from build123d import *

# Parameters (mm, degrees)
F0_W     = 90
F0_H     = 40
F1_DEPTH = 90
F2_ANGLE = 90
F3_W     = 86
F3_H     = 20
F4_DEPTH = 40.001
F5_W     = 36
F5_H     = 20
F6_DEPTH = 90.001


# Not quite as in the source:
# - a feature names something its author has since deleted; it is built from what else it names


with BuildPart() as f1:
    # F0 (on Top) → F1 (new body)
    with BuildSketch(Plane.XY):
        with Locations((-1.7447127029, -1.7198646705)):
            Rectangle(F0_W, F0_H)
    extrude(amount=F1_DEPTH)


with BuildPart() as f1_1:
    # F2: moved
    add(f1.part.rotate(Axis((43.2552872971, 18.2801353295, 45), (0, 0, -1)), F2_ANGLE))

    # F3 (on face) → F4 (cut, through all)
    with BuildSketch(Plane.YZ.offset(43.2552872971)):
        with Locations((63.2801353295, 78)):
            Rectangle(F3_W, F3_H)
        with Locations((63.2801353295, 56)):
            Rectangle(F3_W, F3_H)
        with Locations((63.2801353295, 34)):
            Rectangle(F3_W, F3_H)
        with Locations((63.2801353295, 12)):
            Rectangle(F3_W, F3_H)
    extrude(amount=-F4_DEPTH, mode=Mode.SUBTRACT)

    # F5 (on face) → F6 (cut, through all)
    with BuildSketch(Plane.XZ.offset(-18.2801353295)):
        with Locations((23.2552872971, 78)):
            Rectangle(F5_W, F5_H)
        with Locations((23.2552872971, 56)):
            Rectangle(F5_W, F5_H)
        with Locations((23.2552872971, 34)):
            Rectangle(F5_W, F5_H)
        with Locations((23.2552872971, 12)):
            Rectangle(F5_W, F5_H)
    extrude(amount=-F6_DEPTH, mode=Mode.SUBTRACT)


solid = f1_1.part
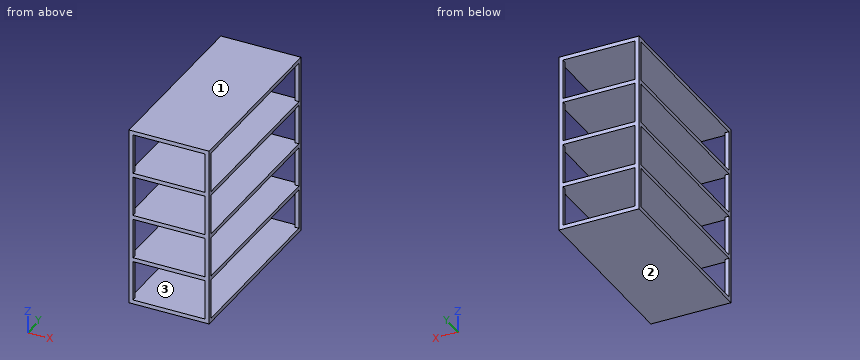
Read the model definition and answer for the solid it produces. Units are mm, in the model's axes. Face numbers are marked on the shaded views. Round coordinates to 2 decimals unless told otherwise and drop trailing zeros. Write each loop counter-clockwise with the first axis right and the second up, starting at its lowest first coordinate (ties: lowest second). Pieces come first, ordered by that corner, then holes.
Q1. Find section B-B on y = 38.5. Determine the outline of the cut face in (x, z), and give its area (3 significant figures).
Values:
outline: (3.26, 0) - (43.26, 0) - (43.26, 2) - (3.26, 2) - close; (3.26, 22) - (43.26, 22) - (43.26, 24) - (3.26, 24) - close; (3.26, 44) - (43.26, 44) - (43.26, 46) - (3.26, 46) - close; (3.26, 66) - (43.26, 66) - (43.26, 68) - (3.26, 68) - close; (3.26, 88) - (43.26, 88) - (43.26, 90) - (3.26, 90) - close
area: 400 mm2
Q2. Find section C-C on z = 84. Determine the outline of the cut face in (x, y).
Values:
outline: (3.26, 18.28) - (5.26, 18.28) - (5.26, 20.28) - (3.26, 20.28) - close; (3.26, 106.28) - (5.26, 106.28) - (5.26, 108.28) - (3.26, 108.28) - close; (41.26, 18.28) - (43.26, 18.28) - (43.26, 20.28) - (41.26, 20.28) - close; (41.26, 106.28) - (43.26, 106.28) - (43.26, 108.28) - (41.26, 108.28) - close
Q3. A straight line is drawn through the part: line 1 (Z direction, x = 18.5, y = 94.5). Find the intervals that lie inside material, in ascending order.
Values:
line 1: z = 0 to 2, 22 to 24, 44 to 46, 66 to 68, 88 to 90
Q4. The mould has two halves that part along Z. Classify the marked faces 1, 2 and 3: released by +Z, released by -Z, zero draft, split by the parting line, or undercut.
Values:
face 1: released by +Z
face 2: released by -Z
face 3: undercut
Q5. Find section A-A on x = 36. Determine the outline of the cut face in (y, z), and give its area (3 significant figures).
Values:
outline: (18.28, 0) - (108.28, 0) - (108.28, 2) - (18.28, 2) - close; (18.28, 22) - (108.28, 22) - (108.28, 24) - (18.28, 24) - close; (18.28, 44) - (108.28, 44) - (108.28, 46) - (18.28, 46) - close; (18.28, 66) - (108.28, 66) - (108.28, 68) - (18.28, 68) - close; (18.28, 88) - (108.28, 88) - (108.28, 90) - (18.28, 90) - close
area: 900 mm2
